Autodesk Inventor part; units mm, degrees
ref_plane "YZ Plane" through (0, 0, 0) normal (1, 0, 0) x (0, 1, 0)
ref_plane "XZ Plane" through (0, 0, 0) normal (0, 1, 0) x (-1, 0, 0)
ref_plane "XY Plane" through (0, 0, 0) normal (0, 0, 1) x (1, 0, 0)
sketch "Sketch1" plane through (0, 0, 0) normal (1, 0, 0) x (0, 1, 0)
  line L0 (5, 0) -> (5, -5.3)
  line L1 (5, -106.9) -> (5, -112.2)
  line L2 (5, -112.2) -> (0, -112.2)
  line L3 (0, -112.2) -> (0, 0)
  line L4 (0, 0) -> (5, 0)
  line L5 (5, -106.9) -> (6, -106.9)
  line L6 (6, -106.9) -> (6, -5.3)
  line L7 (6, -5.3) -> (5, -5.3)
  dimension "d2" = 5
  dimension "d3" = 5.3
  dimension "d4" = 5.3
  dimension "d6" = 112.2
  dimension "d16" = 6
  dimension "d17" = 5
revolve "Revolution1" add sketch "Sketch1" angle 360 about axis through (0, 0, -112.2) along (0, 0, 1)
ref_plane "Work Plane1" through (0, 0, -74.4) normal (0, -1, 0) x (1, 0, 0)
sketch "Sketch3" plane through (0, 0, -74.4) normal (0, -1, 0) x (1, 0, 0)
  circle A0 centre (0, -22.2) radius 2.65
  line L0 (-5, -37.8) -> (5, -37.8)
  line L1 (0, -22.2) -> (0, -37.8) construction
  point P0 (0, 74.4)
  dimension "d12" = 5.3
  dimension "d13" = 15.6
extrude "Extrusion2" cut sketch "Sketch3" along normal blind 10
ref_plane "Work Plane4" through (0, 0, -8.2) normal (0, 0, 1) x (1, 0, 0)
sketch "Sketch5" plane through (-142.34, -16.1386, -8.2) normal (0, 0, 1) x (-0.9033, 0.429, 0)
  line L0 (-121.6494, -68.3151) -> (-115.2993, -71.9814)
  line L1 (-115.2993, -71.9814) -> (-115.2993, -79.3139)
  line L2 (-115.2993, -79.3139) -> (-121.6494, -82.9801)
  line L3 (-121.6494, -82.9801) -> (-127.9995, -79.3139)
  line L4 (-127.9995, -79.3139) -> (-127.9995, -71.9814)
  line L5 (-127.9995, -71.9814) -> (-121.6494, -68.3151)
  line L6 (-121.6494, -82.9801) -> (-121.6494, -68.3151) construction
  point P0 (-121.6494, -75.6476)
  point P1 (-121.6494, -75.6476)
  dimension "d21" = 14.665
extrude "Extrusion4" add sketch "Sketch5" against normal blind 57.15
properties part number "Mecanum Axle" material "Stainless Steel"
CAD build for the part. Positions are in the model's coordinates, mm. A direction names the side the tool comes from. Give positions to 0.01 mm unless a question says otherwise; leave off trailing zeros. Loops run counter-clockwise (first coordinate to the right, second up) from the corner with the lowest first, then second, coordinate; pieces in that order, holes last. Notation, with made-up numbers: M 41,-21 L 85,-21 A23 ccw 85,4 Z; hole C 50,45 d1. An arc over 180 degrees is marked long. Use one line per item in the form item = value.
Item 1: Slice it at B-B (x = 0). List the corners of the cut face in (y, z), plus the area to 3 significant figures.
Determined:
outline = M -6.36,-65.35 L -6,-65.35 L -6,-93.95 L 0,-93.95 L 0,-99.25 L -6,-99.25 L -6,-106.9 L -5,-106.9 L -5,-112.2 L 5,-112.2 L 5,-106.9 L 6,-106.9 L 6,-65.35 L 6.38,-65.35 L 6.38,-8.2 L 6,-8.2 L 6,-5.3 L 5,-5.3 L 5,0 L -5,0 L -5,-5.3 L -6,-5.3 L -6,-8.2 L -6.36,-8.2 Z
area = 1,340 mm2
Item 2: Two-plate mould, pull along Z, no slides. Class faces 4 (the face through (0, 0, -112.2)), 5 (the face through (-0.561, 6.332, -36.375)), 6 (the face through (0, 0, -97)): pulls with the +Z half, pulls with the -Z half, needs draft (parallel to the pull), parting line crosses it, or undercut.
Determined:
face_4 = pulls with the -Z half
face_5 = needs draft
face_6 = undercut
Item 3: Drill centre lines: probe 1 along Z at (x, y) = (0, -2); probe 2 along Z at (x, y) = (-6.5, 0.5); probe 3 along X at (y, z) = (-4.5, -96.6). Where is each one in solid material? Low to high. Write a range as from..to.
Determined:
probe_1 = -112.2..-99.25, -93.95..0
probe_2 = -65.35..-8.2
probe_3 = -3.97..-2.65, 2.65..3.97
Item 4: Slice it at A-A (y = -4). List the corners of the cut face in (x, z), plus the area to 3 significant figures.
Determined:
outline = M -4.95,-65.35 L -4.47,-65.35 L -4.47,-106.9 L -3,-106.9 L -3,-112.2 L 3,-112.2 L 3,-106.9 L 4.47,-106.9 L 4.47,-65.35 L 5.13,-65.35 L 5.13,-8.2 L 4.47,-8.2 L 4.47,-5.3 L 3,-5.3 L 3,0 L -3,0 L -3,-5.3 L -4.47,-5.3 L -4.47,-8.2 L -4.95,-8.2 Z; hole C 0,-96.6 d5.3
area = 1,020 mm2
Item 5: Slice it at D-D (z = -71). List the corners of the cut face in (x, y), plus the area to 3 significant figures.
Determined:
outline = C 0,0 d12
area = 113 mm2
Item 6: Slice it at C-C (y = 1.75). List the corners of the cut face in (x, z).
Determined:
outline = M -6.2,-65.35 L -5.74,-65.35 L -5.74,-106.9 L -4.68,-106.9 L -4.68,-112.2 L 4.68,-112.2 L 4.68,-106.9 L 5.74,-106.9 L 5.74,-65.35 L 6.51,-65.35 L 6.51,-8.2 L 5.74,-8.2 L 5.74,-5.3 L 4.68,-5.3 L 4.68,0 L -4.68,0 L -4.68,-5.3 L -5.74,-5.3 L -5.74,-8.2 L -6.2,-8.2 Z
Item 7: Which spindle directions (+Z, -Z, +X, -X, +Y, -Y) get a long thin tool onto all of the face, cutting with end or side? Do faces 1 (the face through (2, 6, -65.35)), 2 (the face through (-4, -4, -5.3)), 3 (the face through (-0.34, -2.96, -99.23)). Say none if no direction does.
Determined:
face_1 = -Z
face_2 = +Z
face_3 = -Y
Item 8: Flat gauge pins, fed straight in: pin 1 (1 mm diameter, centred on x = -4, y = 4, fed in from -Z); pin 2 (1.5 mm diameter, centred on y = -0.5, z = -91, fed in from +X); pin 3 (6 mm diameter, centred on x = 0, z = -96.6, fed in from -Y). Where does each tip first touch, or does it go through?
Determined:
pin_1 = -106.9
pin_2 = 6
pin_3 = -6
